from build123d import *

# Parameters (mm, degrees)
F1_DEPTH = 1.5875
F2_R     = 19.04999
F3_R     = 6.35
F4_R     = 15.875
F5_DEPTH = 25.4
F6_W     = 63.5
F6_H     = 6.35
F7_DEPTH = 25.4
F8_R     = 1.5875


# Not quite as in the source:
# - a fillet or chamfer is up to 0.001 mm smaller than in the source, because OpenCascade refuses the exact size


with BuildPart() as f1:
    # F0 (on Right) → F1 (new body)
    with BuildSketch(Plane.YZ):
        Polygon((-63.1363113923, 43.5325428513), (-101.2363113923, 43.5325428513), (-101.2363113923, 5.4325428513), (57.5136886077, 5.4325428513), (57.5136886077, -13.6174602094), (63.8636886077, -13.6174602094), (63.8636886077, 18.1325428513), (-63.1363113923, 18.1325428513), align=None)
    extrude(amount=F1_DEPTH)

    # F2 (radius 19.05 in the source; OpenCascade refuses exactly that, so slightly less here)
    f2_edges = [f1.edges().sort_by_distance(p)[0] for p in [
        (0.79375, -63.136311, 43.532543),
        (0.79375, -101.236311, 43.532543),
        (0.79375, -101.236311, 5.432543),
    ]]
    fillet(f2_edges, radius=F2_R)

    # F3
    f3_edges = [f1.edges().sort_by_distance(p)[0] for p in [
        (0.79375, -63.136311, 18.132543),
    ]]
    fillet(f3_edges, radius=F3_R)

    # F4 (on face) → F5 (cut)
    with BuildSketch(Plane.YZ.offset(1.5875)):
        with Locations((-82.1863113923, 24.4825428513)):
            Circle(F4_R)
    extrude(amount=-F5_DEPTH, mode=Mode.SUBTRACT)

    # F6 (on face) → F7 (cut)
    with BuildSketch(Plane.YZ.offset(1.5875)):
        with Locations((19.4136886077, 11.7825428513)):
            Rectangle(F6_W, F6_H)
    extrude(amount=-F7_DEPTH, mode=Mode.SUBTRACT)

    # F8
    f8_edges = [f1.edges().sort_by_distance(p)[0] for p in [
        (0.79375, -12.336311, 14.957543),
        (0.79375, -12.336311, 8.607543),
        (0.79375, 51.163689, 8.607543),
        (0.79375, 51.163689, 14.957543),
    ]]
    fillet(f8_edges, radius=F8_R)


solid = f1.part
Build history of the part. All positions in model axes, mm. Give positions to 0.01 mm unless a question says otherwise; leave off trailing zeros. Loops run counter-clockwise (first coordinate to the right, second up) from the corner with the lowest first, then second, coordinate; pieces in that order, holes last. Notation, with made-up numbers: (25.5, 40.5) -> (74.5, 40.5) arc R25 ccw to (74.5, 70.5) -> close; hole circle Ø4 at (38.5, 15). An arc over 180 degrees is marked (long way). Answer in a Markdown table with one row per item.
Item 1: Probe line 1 along Z through (x, y) = (0.8, 28.5); line 2 along Y through (x, z) = (1.45, 25.5); line 3 along Y through (x, z) = (0.2, 12.5). List the from-to ranges inside material, lowest first. Write a range as [from, to].
Findings below:
| item | result |
|---|---|
| line 1 | z = [5.43, 8.61], [14.96, 18.13] |
| line 2 | y = [-101.21, -98.03], [-66.34, -63.16] |
| line 3 | y = [-97, -92.6], [-71.77, -12.34], [51.16, 63.86] |
Item 2: Slice it at D-D on y = -47. Write the cut outline in (x, z), plus the area to 3 significant figures.
Findings below:
| item | result |
|---|---|
| outline | (0, 5.43) -> (1.59, 5.43) -> (1.59, 18.13) -> (0, 18.13) -> close |
| area | 20.2 mm² |
Item 3: Slice it at B-B on z = 33.5. Write the cut outline in (x, y), plus the area to 3 significant figures.
Findings below:
| item | result |
|---|---|
| outline | (0, -98.97) -> (1.59, -98.97) -> (1.59, -95.25) -> (0, -95.25) -> close; (0, -69.12) -> (1.59, -69.12) -> (1.59, -65.41) -> (0, -65.41) -> close |
| area | 11.8 mm² |
Item 4: Slice it at C-C on x = 1.05. Give the number of separate pieces and of enclosed holes in the cut face, plus the area to 3 significant figures.
Findings below:
| item | result |
|---|---|
| separate pieces | 1 |
| enclosed holes | 2 |
| area | 1,770 mm² |
Item 5: Flat gauge pin, fed straight in: P1, Ø0.8, axis at x = 1, y = 34, coming from the +Z side. Where does the tip first touch, or does it go through?
Findings below:
| item | result |
|---|---|
| P1 | stops at z = 18.13 |
Item 6: Slice it at A-A on y = -9. Write the cut outline in (x, z), plus the area to 3 significant figures.
Findings below:
| item | result |
|---|---|
| outline | (0, 5.43) -> (1.59, 5.43) -> (1.59, 8.61) -> (0, 8.61) -> close; (0, 14.96) -> (1.59, 14.96) -> (1.59, 18.13) -> (0, 18.13) -> close |
| area | 10.1 mm² |
Item 7: Mould opens along Z. For faces 1 (the cylindrical face through (0.805, -68.865, 38.1)), 2 (the flat face through (1.588, -25, 13)), 3 (the cylindrical face through (0.805, -67.522, 18.402)) say: pulls with the +Z half, pulls with the -Z half, needs draft (parallel to the pull), parting line crosses it, or undercut.
Findings below:
| item | result |
|---|---|
| face 1 | pulls with the +Z half |
| face 2 | needs draft |
| face 3 | undercut |
